from build123d import *

# Parameters (mm, degrees)
SKETCH1_R           = 5
SKETCH1_R_2         = 7.5
BOSS_EXTRUDE1_DEPTH = 5
SKETCH2_R           = 2.5
CUT_EXTRUDE1_DEPTH  = 10


with BuildPart() as part:
    # Sketch1 → Boss-Extrude1 (new, symmetric)
    with BuildSketch(Plane.XY):
        with BuildLine():
            ThreePointArc((-4.889177102, 43.953125), (-4.272856259, 33.288034301), (-6.902367673, 22.933823529))
            ThreePointArc((-6.902367673, 22.933823529), (0, 27.5), (6.902367673, 22.933823529))
            ThreePointArc((6.902367673, 22.933823529), (4.272856259, 33.288034301), (4.889177102, 43.953125))
            ThreePointArc((4.889177102, 43.953125), (0, 40), (-4.889177102, 43.953125))
        make_face()
        with Locations((0, 45)):
            Circle(SKETCH1_R)
        with Locations((0, 20)):
            Circle(SKETCH1_R_2)
        with BuildLine():
            ThreePointArc((-4.985162527, -0.384908537), (-0.192597204, 4.996289255), (5, 0))
            ThreePointArc((5, 0), (4.996289255, -0.192597204), (4.985162527, -0.384908537))
            ThreePointArc((4.985162527, -0.384908537), (5.956670882, 9.189806563), (7.387650492, 18.706701807))
            ThreePointArc((7.387650492, 18.706701807), (0, 12.5), (-7.387650492, 18.706701807))
            ThreePointArc((-7.387650492, 18.706701807), (-5.956670882, 9.189806563), (-4.985162527, -0.384908537))
        make_face()
        Circle(SKETCH1_R)
    extrude(amount=BOSS_EXTRUDE1_DEPTH, both=True)

    # Sketch2 → Cut-Extrude1 (cut)
    with BuildSketch(Plane(origin=(0, 0, -5), x_dir=(-1, 0, 0), z_dir=(0, 0, -1))):
        Circle(SKETCH2_R)
    extrude(amount=-CUT_EXTRUDE1_DEPTH, mode=Mode.SUBTRACT)


solid = part.part
Here's how the part is built. I have some questions about the finished solid (model axes, mm). Give positions to 0.01 mm unless a question says otherwise; leave off trailing zeros. Order: outer loops, then holes, each group sorted by start corner. A loop starts at its lowest first (then second) coordinate and runs counter-clockwise, first axis right, second up. Notation, with made-up numbers: (62.5, 7) -> (75.5, 7) arc R23 ccw to (75.5, 24) -> close; hole circle Ø8 at (82, 28.5). An arc over 180 degrees is marked (long way). One line per item, written item: value. Start each with the question number.
1. We'd pull the mould along X, two halves only. Please class faces 1 (the face through (0, 50, 0)), 2 (the face through (-7.448, 20.885, 0.07)), 3 (the face through (0.54, -2.44, -0.07)): released by +X, released by -X, zero draft, split by the parting line, or undercut.
2. Imagine slicing it at D-D, the plane y = 45. List the corners of the cut face in (x, z) for me.
3. I need wall thicknesses on probe 1 along Y at (x, z) = (-0.5, -3); probe 2 along Y at (x, z) = (0.75, -0.25); probe 3 along X at (y, z) = (42.5, -3). Which ranges of each line are inside material? Lowest first, please. Write a range as from..to.
4. Imagine slicing it at C-C, the plane y = 0.5. List the corners of the cut face in (x, z) for me.
5. Imagine slicing it at A-A, the plane x = 0. List the corners of the cut face in (y, z) for me, plus the area to 3 significant figures.
6. Will these pins go through, and if not, where does the flat tip stop? pin 1 Ø4 at (x, z) = (-2.5, 4) entering from +Y; pin 2 Ø1 at (x, z) = (3, 0.5) entering from -Y; pin 3 Ø6 at (x, y) = (0, 0) entering from -Z; pin 4 Ø4 at (x, z) = (4, -3.5) entering from -Y.
7. Imagine slicing it at B-B, the plane z = 4. List the corners of the cut face in (x, y) for me (3 decimals), plus the area to 3 significant figures.
Values follow:
1. face 1: split by the parting line
1. face 2: released by -X
1. face 3: undercut
2. outline: (-5, -5) -> (5, -5) -> (5, 5) -> (-5, 5) -> close
3. probe 1: y = -4.97..-2.45, 2.45..49.97
3. probe 2: y = -4.94..-2.38, 2.38..49.94
3. probe 3: x = -4.61..4.61
4. outline: (-5.06, -5) -> (-2.45, -5) -> (-2.45, 5) -> (-5.06, 5) -> close; (2.45, -5) -> (5.06, -5) -> (5.06, 5) -> (2.45, 5) -> close
5. outline: (-5, -5) -> (-2.5, -5) -> (-2.5, 5) -> (-5, 5) -> close; (2.5, -5) -> (50, -5) -> (50, 5) -> (2.5, 5) -> close
5. area: 500 mm2
6. pin 1: stops at y = 49.97
6. pin 2: stops at y = -4.33
6. pin 3: stops at z = -5
6. pin 4: stops at y = -4.58
7. outline: (-7.388, 18.707) arc R200 cw to (-4.985, -0.385) arc R5 ccw to (4.985, -0.385) arc R200 cw to (7.388, 18.707) arc R7.5 ccw to (6.902, 22.934) arc R35 cw to (4.889, 43.953) arc R5 ccw (long way) to (-4.889, 43.953) arc R35 cw to (-6.902, 22.934) arc R7.5 ccw to start; hole circle Ø5 at (0, 0)
7. area: 560 mm2
